```python
from build123d import *

# Parameters (mm, degrees)
F0_W          = 1366.8883
F0_H          = 38.1
F1_DEPTH      = 38.1
F2_W          = 34.798
F2_H          = 34.798
F3_DEPTH      = 683.44515
F3_DEPTH_BACK = 683.44515
F5_DEPTH      = 38.101


# Not quite as in the source:
# - a feature names something its author has since deleted; it is built from what else it names


with BuildPart() as f1:
    # F0 (on Front) → F1 (new body)
    with BuildSketch(Plane.XZ):
        with Locations((0, -19.05)):
            Rectangle(F0_W, F0_H)
    extrude(amount=F1_DEPTH)

    # F2 (on Right) → F3 (cut, two sides)
    with BuildSketch(Plane.YZ) as f3_sk:
        with Locations((-19.05, -19.05)):
            Rectangle(F2_W, F2_H)
    extrude(amount=-F3_DEPTH, mode=Mode.SUBTRACT)
    extrude(f3_sk.sketch, amount=F3_DEPTH_BACK, mode=Mode.SUBTRACT)

    # F4 (on face) → F5 (cut, through all)
    with BuildSketch(Plane.XZ.offset(38.1)):
        Polygon((649.1544057584, 0), (683.44415, -38.1), (683.44415, 0), align=None)
        Polygon((-683.44415, 0), (-683.44415, -38.1), (-641.1108166729, 0), align=None)
    extrude(amount=-F5_DEPTH, mode=Mode.SUBTRACT)


solid = f1.part
```
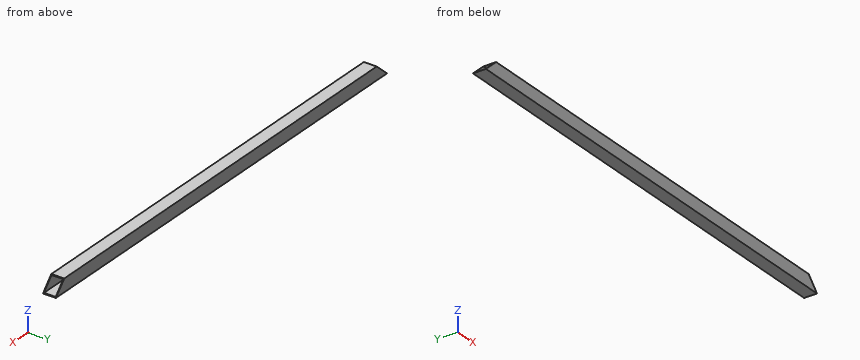
Build history of the part. All positions in model axes, mm. Give positions to 0.01 mm unless a question says otherwise; leave off trailing zeros. Loops run counter-clockwise (first coordinate to the right, second up) from the corner with the lowest first, then second, coordinate; pieces in that order, holes last.
Item 1: Flat gauge pins, fed straight in: pin 1 (10 mm diameter, centred on y = -4.5, z = -22, fed in from -X); pin 2 (12 mm diameter, centred on y = -5, z = -5.5, fed in from -X). Where does each tip first touch, or does it go through?
Answers follow:
pin 1: stops at x = -670.12
pin 2: stops at x = -652.75
Item 2: Slice it at C-C, the plane x = -204. List the corners of the cut face in (y, z), and give its area (3 significant figures).
Answers follow:
outline: (-38.1, -38.1) - (0, -38.1) - (0, 0) - (-38.1, 0) - close; hole (-36.45, -36.45) - (-1.65, -36.45) - (-1.65, -1.65) - (-36.45, -1.65) - close
area: 241 mm2
Item 3: Slice it at A-A, the plane y = -13. List the corners of the cut face in (x, z).
Answers follow:
outline: (-683.44, -38.1) - (683.44, -38.1) - (681.96, -36.45) - (-681.61, -36.45) - close; (-642.95, -1.65) - (650.64, -1.65) - (649.15, 0) - (-641.11, 0) - close
Item 4: Drill centre lines: line 1 (Z direction, x = -580.5, y = -12.5); line 2 (X direction, y = -16, z = -1.5). Where is each one in solid material? Low to high.
Answers follow:
line 1: z = -38.1 to -36.45, -1.65 to 0
line 2: x = -642.78 to 650.5
Item 5: Slice it at B-B, the plane z = -23.5. List the corners of the cut face in (x, y), and give its area (3 significant figures).
Answers follow:
outline: (-667.22, -38.1) - (670.3, -38.1) - (670.3, -36.45) - (-667.22, -36.45) - close; (-667.22, -1.65) - (670.3, -1.65) - (670.3, 0) - (-667.22, 0) - close
area: 4,420 mm2
